from build123d import *

# Parameters (mm, degrees)
BOSS_EXTRUDE6_DEPTH     = 165
CUT_EXTRUDE3_DEPTH      = 381.566986876
CUT_EXTRUDE3_DEPTH_BACK = 381.566986876
SHELL1_T                = -10
SKETCH8_W               = 113
SKETCH8_H               = 116
SKETCH8_W_2             = 107
SKETCH8_H_2             = 110
BOSS_EXTRUDE5_DEPTH     = 4
SKETCH4_RX              = 165
SKETCH4_RY              = 60
BOSS_EXTRUDE7_DEPTH     = 8
SKETCH9_R               = 4
CUT_EXTRUDE4_DEPTH      = 10
SCALE1_SCALE            = 0.5


with BuildPart() as part:
    # Sketch1 → Revolve1 (revolve)
    with BuildSketch(Plane.XY, mode=Mode.PRIVATE) as revolve1_sk:
        Polygon((240, 0), (213.550952894, 150), (0, 150), (0, 0), (0, -30), (180, -30), (193.356860559, 0), align=None)
    revolve(revolve1_sk.sketch.rotate(Axis((0, 150, 0), (0, -1, 0)), 180), axis=Axis((0, 150, 0), (0, -1, 0)))

    # Sketch2 → Boss-Extrude6 (add, symmetric)
    with BuildSketch(Plane.XY):
        Polygon((20, -30), (144.519146375, -30), (249.534028741, -30), (249.534028741, -8), (220.263749943, 158), (20, 158), align=None)
    extrude(amount=BOSS_EXTRUDE6_DEPTH, both=True)

    # Sketch5 → Revolve3 (revolve)
    with BuildSketch(Plane.XY, mode=Mode.PRIVATE) as revolve3_sk:
        Polygon((0, -30), (0, -60), (90, -60), (105, -30), align=None)
    revolve(revolve3_sk.sketch.rotate(Axis((0, -30, 0), (0, -1, 0)), 180), axis=Axis((0, -30, 0), (0, -1, 0)))

    # Sketch7 → Cut-Extrude3 (cut, two sides)
    with BuildSketch(Plane.XY) as cut_extrude3_sk:
        Polygon((149.534028741, 158), (190.922477213, -8), (190.922477213, -30), (249.534028741, -30), (249.534028741, 158), align=None)
    extrude(amount=CUT_EXTRUDE3_DEPTH, mode=Mode.SUBTRACT)
    extrude(cut_extrude3_sk.sketch, amount=-CUT_EXTRUDE3_DEPTH_BACK, mode=Mode.SUBTRACT)

    # Shell1
    shell1_openings = [part.faces().sort_by_distance(p)[0] for p in [
        (0, -60, 0),
    ]]
    offset(amount=SHELL1_T, openings=shell1_openings, kind=Kind.INTERSECTION)

    # Sketch8 → Boss-Extrude5 (add)
    with BuildSketch(Plane(origin=(177.870623194, 44.348127245, 0), x_dir=(0, 0, -1), z_dir=(0.9702957262759971, 0.24192189559966487, 0))):
        with Locations((-78.5, 15)):
            Rectangle(SKETCH8_W, SKETCH8_H)
        with Locations((-78.5, 15)):
            Rectangle(SKETCH8_W_2, SKETCH8_H_2, mode=Mode.SUBTRACT)
        with Locations((78.5, 15)):
            Rectangle(SKETCH8_W, SKETCH8_H)
        with Locations((78.5, 15)):
            Rectangle(SKETCH8_W_2, SKETCH8_H_2, mode=Mode.SUBTRACT)
    extrude(amount=BOSS_EXTRUDE5_DEPTH)

    # Sketch4 → Boss-Extrude7 (add)
    with BuildSketch(Plane(origin=(0, 150, 0), x_dir=(1, 0, 0), z_dir=(0, 1, 0))):
        with Locations(Location((20, 0), (0, 0, 90))):
            Ellipse(SKETCH4_RX, SKETCH4_RY)
    extrude(amount=BOSS_EXTRUDE7_DEPTH)

    # Sketch9 → Cut-Extrude4 (cut)
    with BuildSketch(Plane(origin=(177.870623194, 44.348127245, 0), x_dir=(0, 0, -1), z_dir=(0.9702957262759971, 0.24192189559966487, 0))):
        with Locations(Location((-120, 88, 0), (0, 0, 90))):
            Circle(SKETCH9_R)
    cut_extrude4 = extrude(amount=-CUT_EXTRUDE4_DEPTH, mode=Mode.SUBTRACT)

    # Mirror1: Cut-Extrude4 across plane
    add(cut_extrude4.mirror(Plane.XY), mode=Mode.SUBTRACT)


with BuildPart() as part_1:
    # Scale1: scaled about (0, 0, 0)
    add(part.part.scale(SCALE1_SCALE))


solid = part_1.part
For this review, take the finished solid that the model builds, in its own axes (mm). A direction names the side the tool comes from. Round coordinates to 2 decimals unless told otherwise and drop trailing zeros. Order: outer loops, then holes, each group sorted by start corner. A loop starts at its lowest first (then second) coordinate and runs counter-clockwise, first axis right, second up. Notation, with made-up numbers: (3, 57.25) -> (55, 57.25) arc R25 ccw to (55, 69.25) -> close; hole circle Ø10 at (69.25, 29). An arc over 180 degrees is marked (long way). Write item = value, one per line. Start each with the question number.
1) The part is to be moulded in two halves that separate along Y. For faces 1 (the face through (90.461, -7, 1)), 2 (the face through (0, -30, 40)), 3 (the face through (-110.295, 54.692, 3.682)), 4 (the face through (88, 29, -11)), say which applies: +Y half, -Y half, draft (parallel to the pull), parting line (faces both ways), or undercut.
2) Tool access review of faces 5 (the face through (95.461, -9, 1)), 6 (the face through (88, 29, 11)), 7 (the face through (81, 29, -82.5)), 8 (the face through (88, 29, -67.5)), 9 (the face through (81, 20, -77.5)): name each direction out of +Z, -Z, +X, -X, +Y, -Y from which nothing blocks a thin tool from reaching the whole face with its end or side.
3) To check wall thickness, follow line 1 (Y direction, x = 62, z = 64.5); line 2 (Y direction, x = -65, z = 7); line 3 (Z direction, x = -67, y = 54.5). State the ranges of each line that lie inside material, in increasing order. Write a range as from..to.
4) Take a section at A-A on y = 38. State the section outline as (x, z) points.
5) Insertion check: pin 1 (8 mm diameter, centred on x = -32, z = -32.5, fed in from +Y); pin 2 (12 mm diameter, centred on x = 90.5, y = 43, fed in from +Z); pin 3 (17 mm diameter, centred on x = 88.5, y = 27, fed in from -Z). Each pin has a flat end and moves straight along its axis. Give the tip position at first contact, or say it passes through.
Verdict:
q1.face_1 = undercut
q1.face_2 = -Y half
q1.face_3 = +Y half
q1.face_4 = draft
q2.face_5 = +Z, -Z, +X, -Y
q2.face_6 = +X, +Y
q2.face_7 = -Z, +X
q2.face_8 = -Z, +X, +Y
q2.face_9 = none
q3.line_1 = -15..-10, 74..79
q3.line_2 = -15..-10, 70..75
q3.line_3 = -87.73..-81.25, 81.25..87.73
q4.outline = (77.66, -82.5) -> (84.99, -82.5) -> (84.99, -67.5) -> (87.05, -67.5) -> (87.05, -66) -> (84.99, -66) -> (84.99, -12.5) -> (87.05, -12.5) -> (87.05, -11) -> (84.99, -11) -> (84.99, 11) -> (87.05, 11) -> (87.05, 12.5) -> (84.99, 12.5) -> (84.99, 66) -> (87.05, 66) -> (87.05, 67.5) -> (84.99, 67.5) -> (84.99, 82.5) -> (77.66, 82.5) arc R113.3 ccw (long way) to start; hole (75.54, -77.5) -> (79.84, -77.5) -> (79.84, 77.5) -> (75.54, 77.5) arc R108.22 ccw (long way) to start
q5.pin_1 = 75
q5.pin_2 = 67.5
q5.pin_3 = -83.21
